Source: CAD feature listing. Evaluate the final solid. Frame: model axes, mm. Face numbers are marked on the shaded views. A direction names the side the tool comes from. Give positions to 0.01 mm unless a question says otherwise; leave off trailing zeros. Loops run counter-clockwise (first coordinate to the right, second up) from the corner with the lowest first, then second, coordinate; pieces in that order, holes last.
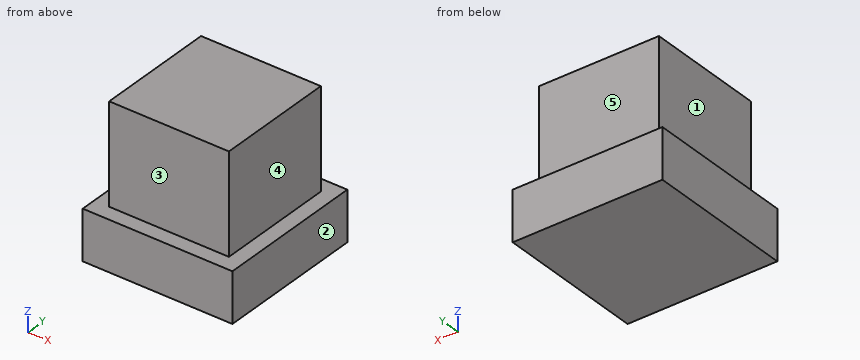
from build123d import *

# Parameters (mm, degrees)
F0_W     = 15
F0_H     = 15
F0_W_2   = 12
F0_H_2   = 12
F1_DEPTH = 5
F2_DEPTH = 10


with BuildPart() as f1:
    # F0 (on Top) → F1 (new body)
    with BuildSketch(Plane.XY):
        Rectangle(F0_W, F0_H)
        Rectangle(F0_W_2, F0_H_2, mode=Mode.SUBTRACT)
        Rectangle(F0_W_2, F0_H_2)
    extrude(amount=-F1_DEPTH)

    # F0 (on Top) → F2 (join)
    with BuildSketch(Plane.XY):
        Rectangle(F0_W_2, F0_H_2)
    extrude(amount=F2_DEPTH)


solid = f1.part
1) Ray query, probe 1 along Z at (x, y) = (-3.75, 6.75); probe 2 along X at (y, z) = (-1.75, 7.75). Return the intervals inside material, ascending.
Checks:
probe 1: z = -5 to 0
probe 2: x = -6 to 6
2) Contact query for flat-ended pins moving along their axis: P1, Ø8, axis at y = -2.5, z = 6.5, coming from the -X side; P2, Ø3, axis at x = -1, z = 5, coming from the +Y side; P3, Ø6, axis at y = 1.5, z = 1.5, coming from the +X side; P4, Ø5, axis at x = 0, z = 3, coming from the -Y side. Output: stop coordinate, or through.
Checks:
P1: stops at x = -6
P2: stops at y = 6
P3: stops at x = 7.5
P4: stops at y = -6
3) Reachability of the marked faces 1, 2, 3, 4 and 5 from +Z, -Z, +X, -X, +Y, -Y: full face, straight path, thin tool, end or side. Return the list, or none.
Checks:
face 1: +Z, -X, +Y, -Y
face 2: +Z, -Z, +X, +Y, -Y
face 3: +Z, +X, -X, -Y
face 4: +Z, +X, +Y, -Y
face 5: +Z, +X, -X, +Y
4) Cut plane A-A (y = 1). Return loops of the section in (x, z).
Checks:
outline: (-7.5, -5) - (7.5, -5) - (7.5, 0) - (6, 0) - (6, 10) - (-6, 10) - (-6, 0) - (-7.5, 0) - close
5) Cut plane C-C (z = 5.75). Return loops of the section in (x, y), and give its area (3 significant figures).
Checks:
outline: (-6, -6) - (6, -6) - (6, 6) - (-6, 6) - close
area: 144 mm2
